CAD build for the part. Positions are in the model's coordinates, mm. Coordinates: 2 decimals unless noted, no trailing zeros. Order: outer loops, then holes, each group sorted by start corner. A loop starts at its lowest first (then second) coordinate and runs counter-clockwise, first axis right, second up. Notation, with made-up numbers: M 33,-36 L 37,-36 A28 cw 37,-5 Z; hole C 40.25,2.25 d11. An arc over 180 degrees is marked long. Write item = value, one per line.
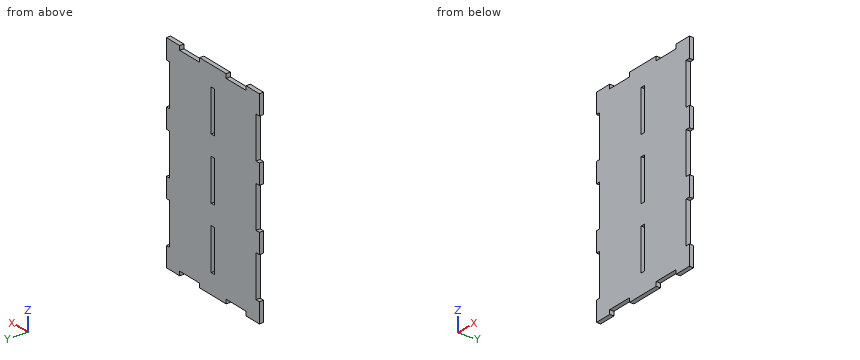
Autodesk Inventor part; units mm, degrees
ref_plane "YZ Plane" through (0, 0, 0) normal (1, 0, 0) x (0, 1, 0)
ref_plane "XZ Plane" through (0, 0, 0) normal (0, 1, 0) x (-1, 0, 0)
ref_plane "XY Plane" through (0, 0, 0) normal (0, 0, 1) x (1, 0, 0)
sketch "Sketch1" plane through (0, 0, 0) normal (0, 1, 0) x (-1, 0, 0)
  line L0 (0, 0) -> (-140, 0)
  line L1 (-140, 0) -> (-140, 245)
  line L2 (-140, 245) -> (0, 245)
  line L3 (0, 245) -> (0, 0)
  dimension "d0" = 140
  dimension "d1" = 245
extrude "Extrusion1" add sketch "Sketch1" along normal blind 5
sketch "Sketch2" plane through (0, 5, 0) normal (0, 1, 0) x (1, 0, 0)
  line L0 (0, -245) -> (140, -245)
  line L1 (140, -245) -> (140, 0)
  line L2 (140, 0) -> (0, 0)
  line L3 (0, 0) -> (0, -245)
  line L4 (135, -73.75) -> (140, -73.75)
  line L5 (140, -73.75) -> (140, -23.75)
  line L6 (140, -23.75) -> (135, -23.75)
  line L7 (135, -23.75) -> (135, -73.75)
  line L8 (135, -221.25) -> (140, -221.25)
  line L9 (140, -221.25) -> (140, -171.25)
  line L10 (140, -171.25) -> (135, -171.25)
  line L11 (135, -171.25) -> (135, -221.25)
  line L12 (135, -147.5) -> (140, -147.5)
  line L13 (140, -147.5) -> (140, -97.5)
  line L14 (140, -97.5) -> (135, -97.5)
  line L15 (135, -97.5) -> (135, -147.5)
  line L16 (0, -73.75) -> (5, -73.75)
  line L17 (5, -73.75) -> (5, -23.75)
  line L18 (5, -23.75) -> (0, -23.75)
  line L19 (0, -23.75) -> (0, -73.75)
  line L20 (0, -221.25) -> (5, -221.25)
  line L21 (5, -221.25) -> (5, -171.25)
  line L22 (5, -171.25) -> (0, -171.25)
  line L23 (0, -171.25) -> (0, -221.25)
  line L24 (0, -147.5) -> (5, -147.5)
  line L25 (5, -147.5) -> (5, -97.5)
  line L26 (5, -97.5) -> (0, -97.5)
  line L27 (0, -97.5) -> (0, -147.5)
  line L28 (20, -245) -> (50, -245)
  line L29 (50, -245) -> (50, -240)
  line L30 (50, -240) -> (20, -240)
  line L31 (20, -240) -> (20, -245)
  line L32 (90, -245) -> (120, -245)
  line L33 (120, -245) -> (120, -240)
  line L34 (120, -240) -> (90, -240)
  line L35 (90, -240) -> (90, -245)
  line L36 (20, -5) -> (50, -5)
  line L37 (50, -5) -> (50, 0)
  line L38 (50, 0) -> (20, 0)
  line L39 (20, 0) -> (20, -5)
  line L40 (120, 0) -> (90, 0)
  line L41 (90, 0) -> (90, -5)
  line L42 (90, -5) -> (120, -5)
  line L43 (120, -5) -> (120, 0)
  point P0 (140, -23.75)
  dimension "d4" = 50
  dimension "d5" = 5
  dimension "d6" = 50
  dimension "d7" = 5
  dimension "d8" = 50
  dimension "d9" = 5
  dimension "d10" = 23.75
  dimension "d11" = 23.75
  dimension "d12" = 23.75
  dimension "d13" = 50
  dimension "d14" = 5
  dimension "d15" = 50
  dimension "d16" = 5
  dimension "d17" = 50
  dimension "d18" = 5
  dimension "d19" = 23.75
  dimension "d20" = 23.75
  dimension "d21" = 23.75
  dimension "d22" = 20
  dimension "d23" = 5
  dimension "d25" = 30
  dimension "d26" = 5
  dimension "d27" = 30
  dimension "d28" = 5
  dimension "d29" = 30
  dimension "d30" = 5
  dimension "d31" = 30
  dimension "d32" = 20
  dimension "d33" = 20
  dimension "d34" = 20
extrude "Extrusion2" cut sketch "Sketch2" against normal blind 5 contours L31 L30 L29 L0 | L3 L22 L21 L20 | L35 L34 L33 L0 | L3 L26 L25 L24 | L3 L18 L17 L16 | L8 L11 L10 L1 | L12 L15 L14 L1 | L2 L37 L36 L39 | L4 L7 L6 L1 | L2 L43 L42 L41
sketch "Sketch3" plane through (0, 5, 0) normal (0, 1, 0) x (1, 0, 0)
  line L0 (0, -147.5) -> (5, -147.5)
  line L1 (5, -147.5) -> (5, -97.5)
  line L2 (5, -97.5) -> (0, -97.5)
  line L3 (0, -73.75) -> (0, -97.5)
  line L4 (0, -73.75) -> (5, -73.75)
  line L5 (5, -73.75) -> (5, -23.75)
  line L6 (5, -23.75) -> (0, -23.75)
  line L7 (0, 0) -> (0, -23.75)
  line L8 (20, 0) -> (0, 0)
  line L9 (20, 0) -> (20, -5)
  line L10 (20, -5) -> (50, -5)
  line L11 (50, -5) -> (50, 0)
  line L12 (90, 0) -> (50, 0)
  line L13 (90, 0) -> (90, -5)
  line L14 (90, -5) -> (120, -5)
  line L15 (120, -5) -> (120, 0)
  line L16 (140, 0) -> (120, 0)
  line L17 (140, -23.75) -> (140, 0)
  line L18 (140, -23.75) -> (135, -23.75)
  line L19 (135, -23.75) -> (135, -73.75)
  line L20 (135, -73.75) -> (140, -73.75)
  line L21 (140, -97.5) -> (140, -73.75)
  line L22 (140, -97.5) -> (135, -97.5)
  line L23 (135, -97.5) -> (135, -147.5)
  line L24 (135, -147.5) -> (140, -147.5)
  line L25 (140, -171.25) -> (140, -147.5)
  line L26 (140, -171.25) -> (135, -171.25)
  line L27 (135, -171.25) -> (135, -221.25)
  line L28 (135, -221.25) -> (140, -221.25)
  line L29 (140, -245) -> (140, -221.25)
  line L30 (120, -245) -> (140, -245)
  line L31 (120, -245) -> (120, -240)
  line L32 (120, -240) -> (90, -240)
  line L33 (90, -240) -> (90, -245)
  line L34 (50, -245) -> (90, -245)
  line L35 (50, -245) -> (50, -240)
  line L36 (50, -240) -> (20, -240)
  line L37 (20, -240) -> (20, -245)
  line L38 (0, -245) -> (20, -245)
  line L39 (0, -221.25) -> (0, -245)
  line L40 (0, -221.25) -> (5, -221.25)
  line L41 (5, -221.25) -> (5, -171.25)
  line L42 (5, -171.25) -> (0, -171.25)
  line L43 (0, -147.5) -> (0, -171.25)
  line L44 (135, -171.25) -> (135, -221.25) construction
  line L45 (135, -186.5648) -> (72.5, -186.5648) construction
  line L46 (67.5, -245) -> (72.5, -245)
  line L47 (72.5, 0) -> (67.5, 0)
  line L48 (67.5, -221.25) -> (72.5, -221.25)
  line L49 (67.5, -171.25) -> (72.5, -171.25)
  line L50 (67.5, -73.75) -> (72.5, -73.75)
  line L51 (67.5, -23.75) -> (72.5, -23.75)
  line L52 (67.5, -147.5) -> (72.5, -147.5)
  line L53 (67.5, -97.5) -> (72.5, -97.5)
  line L54 (67.5, -171.25) -> (67.5, -221.25)
  line L55 (72.5, -221.25) -> (72.5, -171.25)
  line L56 (72.5, -147.5) -> (72.5, -97.5)
  line L57 (72.5, -73.75) -> (72.5, -23.75)
  line L58 (67.5, -23.75) -> (67.5, -73.75)
  line L59 (67.5, -97.5) -> (67.5, -147.5)
  dimension "d37" = 62.5
  dimension "d39" = 23.75
  dimension "d40" = 50
  dimension "d41" = 23.75
  dimension "d42" = 50
  dimension "d43" = 50
  dimension "d44" = 23.75
  dimension "d45" = 5
extrude "Extrusion3" cut sketch "Sketch3" against normal blind 5 contours L54 L49 L55 L48 | L58 L51 L57 L50 | L59 L53 L56 L52
properties part number "Lateral 1"
(1) Wall check: line 1 (Z direction, x = 68.5, y = 1.7); line 2 (X direction, y = 2.6, z = 203); line 3 (Z direction, x = 30.5, y = 4.6). Give the ranges that are in metal, low to high. Write a range as from..to.
Evaluation:
line_1 = 0..23.75, 73.75..97.5, 147.5..171.25, 221.25..245
line_2 = 5..67.5, 72.5..135
line_3 = 5..240
(2) Pin check, flat tips, straight feed: pin 1 Ø3 at (x, z) = (29, 193.5) entering from -Y; pin 2 Ø2.5 at (y, z) = (3, 48.5) entering from +X; pin 3 Ø1.5 at (y, z) = (3.5, 118) entering from -X. Stop position of each tip, or through.
Evaluation:
pin_1 = 0
pin_2 = 135
pin_3 = 5
(3) Slice it at B-B, the plane y = 2.85. State how many separate pieces and enclosed holes the cut face has, then the cut area to 4 significant figures.
Evaluation:
separate_pieces = 1
enclosed_holes = 3
area = 31,450 mm²
(4) Slice it at A-A, the plane z = 192. Write the cut outline in (x, y), then the cut area to 3 significant figures.
Evaluation:
outline = M 5,0 L 67.5,0 L 67.5,5 L 5,5 Z; M 72.5,0 L 135,0 L 135,5 L 72.5,5 Z
area = 625 mm²
(5) Slice it at C-C, the plane x = 35. Write the cut outline in (y, z), then the cut area to 4 significant figures.
Evaluation:
outline = M 0,5 L 5,5 L 5,240 L 0,240 Z
area = 1,175 mm²
